For this review, take the finished solid that the model builds, in its own axes (mm). A direction names the side the tool comes from. Give positions to 0.01 mm unless a question says otherwise; leave off trailing zeros. Order: outer loops, then holes, each group sorted by start corner. A loop starts at its lowest first (then second) coordinate and runs counter-clockwise, first axis right, second up.
from build123d import *

# Parameters (mm, degrees)
BOSS_EXTRU_1_DEPTH      = 3.5
ESQUISSE2_R             = 2.5
ENL_V_MAT_EXTRU_1_DEPTH = 3.5
ESQUISSE3_W             = 4
ESQUISSE3_H             = 70
BOSS_EXTRU_2_DEPTH      = 60
ESQUISSE4_R             = 8
ENL_V_MAT_EXTRU_2_DEPTH = 6
CONG_1_R                = 30
ESQUISSE5_W             = 3.5
ESQUISSE5_H             = 70
BOSS_EXTRU_4_DEPTH      = 11.5
CONG_3_R                = 7


with BuildPart() as part:
    # Esquisse1 → Boss.-Extru.1 (new body)
    with BuildSketch(Plane.XY):
        with BuildLine():
            Line((9.27027027, 7.756756757), (16.27027027, 7.756756757))
            Line((16.27027027, 7.756756757), (16.27027027, 0.756756757))
            Line((16.27027027, 0.756756757), (16.27027027, -55.243243243))
            Line((16.27027027, -55.243243243), (16.27027027, -62.243243243))
            Line((16.27027027, -62.243243243), (9.27027027, -62.243243243))
            Line((9.27027027, -62.243243243), (3.27027027, -62.243243243))
            ThreePointArc((3.27027027, -62.243243243), (-1.679477198, -60.192990712), (-3.72972973, -55.243243243))
            Line((-3.72972973, -55.243243243), (-3.72972973, 0.756756757))
            ThreePointArc((-3.72972973, 0.756756757), (-1.679477198, 5.706504225), (3.27027027, 7.756756757))
            Line((3.27027027, 7.756756757), (9.27027027, 7.756756757))
        make_face()
    extrude(amount=BOSS_EXTRU_1_DEPTH)

    # Esquisse2 → Enlèv. mat.-Extru.1 (cut)
    with BuildSketch(Plane.XY.offset(3.5)):
        with Locations((6.27027027, -7.243243243)):
            Circle(ESQUISSE2_R)
        with Locations((6.27027027, -47.243243243)):
            Circle(ESQUISSE2_R)
    extrude(amount=-ENL_V_MAT_EXTRU_1_DEPTH, mode=Mode.SUBTRACT)



with BuildPart() as body_2:
    # Esquisse3 → Boss.-Extru.2 (new body)
    with BuildSketch(Plane.XY.offset(3.5)):
        with Locations((25.77027027, -27.243243243)):
            Rectangle(ESQUISSE3_W, ESQUISSE3_H)
    extrude(amount=BOSS_EXTRU_2_DEPTH)

    # Esquisse4 → Enlèv. mat.-Extru.2 (cut)
    with BuildSketch(Plane(origin=(27.77027027, 0, 0), x_dir=(0, 0, -1), z_dir=(1, 0, 0))):
        with Locations(Location((-38.5, -27.243243243, 0), (0, 0, 90))):
            Circle(ESQUISSE4_R)
    extrude(amount=-ENL_V_MAT_EXTRU_2_DEPTH, mode=Mode.SUBTRACT)

    # Congé1
    cong_1_edges = [body_2.edges().sort_by_distance(p)[0] for p in [
        (25.77027027, 7.756756757, 63.5),
        (25.77027027, -62.243243243, 63.5),
    ]]
    fillet(cong_1_edges, radius=CONG_1_R)


with BuildPart() as part_1:
    add(part.part)

    add(body_2.part)  # Boss.-Extru.4 merges body 2
    # Esquisse5 → Boss.-Extru.4 (add)
    with BuildSketch(Plane(origin=(16.27027027, 0, 0), x_dir=(0, 0, -1), z_dir=(1, 0, 0))):
        with Locations((-1.75, -27.243243243)):
            Rectangle(ESQUISSE5_W, ESQUISSE5_H)
    extrude(amount=BOSS_EXTRU_4_DEPTH)

    # Congé3
    cong_3_edges = [part_1.edges().sort_by_distance(p)[0] for p in [
        (23.77027027, -27.243243243, 3.5),
    ]]
    fillet(cong_3_edges, radius=CONG_3_R)


solid = part_1.part
1) We need section C-C on x = 2. Give the boundary of the cut face in (y, z), then the cut area to 3 significant figures.
Answer sheet:
outline: (-62.13, 0) - (7.64, 0) - (7.64, 3.5) - (-62.13, 3.5) - close
area: 244 mm2
2) We need section B-B on y = -41.5. Give the boundary of the cut face in (x, z), then the cut area to 3 significant figures.
Answer sheet:
outline: (-3.73, 0) - (27.77, 0) - (27.77, 62.04) - (23.77, 62.04) - (23.77, 10.5) arc R7 cw to (16.77, 3.5) - (-3.73, 3.5) - close
area: 355 mm2
3) To check wall thickness, follow line 1 (Z direction, x = 12, y = -54.5); line 2 (X direction, y = -22.5, z = 52); line 3 (Y direction, x = 26, z = 38). State the ranges of each line that lie inside material, in increasing order.
Answer sheet:
line 1: z = 0 to 3.5
line 2: x = 23.77 to 27.77
line 3: y = -61.9 to -35.23, -19.26 to 7.42
4) Clearance check with flat-ended pins moving along their axes: pin 1 (10 mm diameter, centred on x = 15, y = -48, fed in from +Z); pin 2 (3 mm diameter, centred on y = -42, z = 51.5, fed in from -X); pin 3 (16.5 mm diameter, centred on x = 1.5, y = -31, fed in from +Z). State where each tip first meets the part, or that it passes through.
Answer sheet:
pin 1: stops at z = 4.29
pin 2: stops at x = 23.77
pin 3: stops at z = 3.5
5) We need section D-D on z = 45. Give the boundary of the cut face in (x, y).
Answer sheet:
outline: (23.77, -59.95) - (27.77, -59.95) - (27.77, -31.91) - (23.77, -31.91) - close; (23.77, -22.58) - (27.77, -22.58) - (27.77, 5.47) - (23.77, 5.47) - close
6) Draft analysis for pull direction Y (two halves, no side actions). For faces 3 (the face through (24, 7.757, 8)), 4 (the face through (5.728, -49.684, 1.774)), 5 (the face through (25.798, -53.688, 54.479)), state which applies: +Y half, -Y half, draft (parallel to the pull), parting line (faces both ways), or undercut.
Answer sheet:
face 3: +Y half
face 4: undercut
face 5: -Y half
7) Tool access review of faces 1 (the face through (-1.734, 5.652, 1.726)), 2 (the face through (23.77, -36, 37)): name each direction out of +Z, -Z, +X, -X, +Y, -Y from which nothing blocks a thin tool from reaching the whole face with its end or side.
Answer sheet:
face 1: +Z, -Z, -X, +Y
face 2: +Z, -X, +Y, -Y
8) We need section A-A on z = 38.5. Give the boundary of the cut face in (x, y), then the cut area to 3 significant figures.
Answer sheet:
outline: (23.77, -61.82) - (27.77, -61.82) - (27.77, -35.24) - (23.77, -35.24) - close; (23.77, -19.24) - (27.77, -19.24) - (27.77, 7.34) - (23.77, 7.34) - close
area: 213 mm2
